from build123d import *

# Parameters (mm, degrees)
SKETCH1_W               = 22
SKETCH1_H               = 28
BOSS_EXTRUDE1_DEPTH     = 1.75
SKETCH2_R               = 1.3
SKETCH2_R_2             = 1
CUT_EXTRUDE1_DEPTH      = 18.890290663
SKETCH3_R               = 0.6
CUT_EXTRUDE2_DEPTH      = 18.890290663
LPATTERN1_COUNT         = 4
LPATTERN1_PITCH         = 2.54
MIRROR1_COPY_1_SKETCH_R = 0.6
MIRROR1_COPY_1_DEPTH    = 18.890290663
MIRROR1_COPY_2_SKETCH_R = 0.6
MIRROR1_COPY_2_DEPTH    = 18.890290663
MIRROR1_COPY_3_SKETCH_R = 0.6
MIRROR1_COPY_3_DEPTH    = 18.890290663
SKETCH4_W               = 5
SKETCH4_H               = 4.4
BOSS_EXTRUDE2_DEPTH     = 1.2


with BuildPart() as part:
    # Sketch1 → Boss-Extrude1 (new body)
    with BuildSketch(Plane.XY):
        Rectangle(SKETCH1_W, SKETCH1_H)
    extrude(amount=BOSS_EXTRUDE1_DEPTH)

    # Sketch2 → Cut-Extrude1 (cut, through all)
    with BuildSketch(Plane.XY.offset(1.75)):
        with Locations((-9, -1)):
            Circle(SKETCH2_R)
        with Locations((-9, -12)):
            Circle(SKETCH2_R)
        with Locations((9, -12)):
            Circle(SKETCH2_R)
        with Locations((9, -1)):
            Circle(SKETCH2_R)
        with Locations((0, -6.5)):
            Circle(SKETCH2_R_2)
    extrude(amount=-CUT_EXTRUDE1_DEPTH, mode=Mode.SUBTRACT)

    # Sketch3 → Cut-Extrude2 (cut, through all)
    with BuildSketch(Plane.XY.offset(1.75)):
        with Locations((-1.27, 12.73)):
            Circle(SKETCH3_R)
    cut_extrude2 = extrude(amount=-CUT_EXTRUDE2_DEPTH, mode=Mode.SUBTRACT)

    # LPattern1: Cut-Extrude2 ×4
    with Locations(*[(-i * LPATTERN1_PITCH, 0, 0) for i in range(1, LPATTERN1_COUNT)]):
        add(cut_extrude2, mode=Mode.SUBTRACT)

    # Mirror1: Cut-Extrude2 across plane
    add(cut_extrude2.mirror(Plane(origin=(0, 0, 0), x_dir=(0, 0, 1), z_dir=(1, 0, 0))), mode=Mode.SUBTRACT)

    # Mirror1 copy 1 sketch → Mirror1 copy 1 (cut, through all)
    with BuildSketch(Plane(origin=(2.54, 0, 1.75), x_dir=(-1, 0, 0), z_dir=(0, 0, 1))):
        with Locations((-1.27, -12.73)):
            Circle(MIRROR1_COPY_1_SKETCH_R)
    extrude(amount=-MIRROR1_COPY_1_DEPTH, mode=Mode.SUBTRACT)

    # Mirror1 copy 2 sketch → Mirror1 copy 2 (cut, through all)
    with BuildSketch(Plane(origin=(5.08, 0, 1.75), x_dir=(-1, 0, 0), z_dir=(0, 0, 1))):
        with Locations((-1.27, -12.73)):
            Circle(MIRROR1_COPY_2_SKETCH_R)
    extrude(amount=-MIRROR1_COPY_2_DEPTH, mode=Mode.SUBTRACT)

    # Mirror1 copy 3 sketch → Mirror1 copy 3 (cut, through all)
    with BuildSketch(Plane(origin=(7.62, 0, 1.75), x_dir=(-1, 0, 0), z_dir=(0, 0, 1))):
        with Locations((-1.27, -12.73)):
            Circle(MIRROR1_COPY_3_SKETCH_R)
    extrude(amount=-MIRROR1_COPY_3_DEPTH, mode=Mode.SUBTRACT)

    # Sketch4 → Boss-Extrude2 (add)
    with BuildSketch(Plane.XY.offset(1.75)):
        with Locations((0, -6.5)):
            Rectangle(SKETCH4_W, SKETCH4_H)
    extrude(amount=BOSS_EXTRUDE2_DEPTH)


solid = part.part
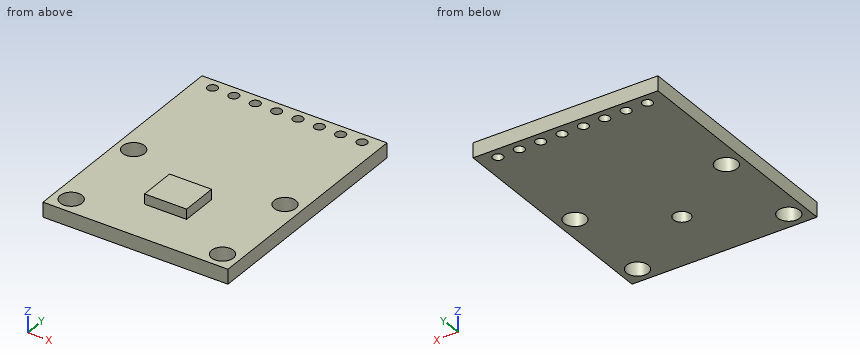
The model under review builds one solid part; all positions refer to its coordinate system, in mm. Give positions to 0.01 mm unless a question says otherwise; leave off trailing zeros. Loops run counter-clockwise (first coordinate to the right, second up) from the corner with the lowest first, then second, coordinate; pieces in that order, holes last. Notation, with made-up numbers: (61, 48) -> (114, 48) arc R25 ccw to (114, 85) -> close; hole circle Ø3 at (49, 74.25). An arc over 180 degrees is marked (long way). Put each result on its own line as item: value. Start each with the question number.
1. We need section D-D on x = -9. State the section outline as (y, z) points.
2. Wall thickness on probe 1 along Y at (x, z) = (9, 0.7); probe 2 along Z at (x, y) = (7.5, -6.5); probe 3 along Y at (x, z) = (1.5, 2.45): over which ranges is each line inside the solid? List them lowest first.
3. We need section C-C on y = -6.5. State the section outline as (x, z) points, then the cut area to 3 significant figures.
4. Clearance check with flat-ended pins moving along their axes: P1, Ø1.9, axis at x = 8.89, y = 12.73, coming from the +Z side; P2, Ø0.6, axis at x = 1, z = 2.5, coming from the +Y side. State where each tip first meets the part, or that it passes through.
5. We need section A-A on x = 6.35. State the section outline as (y, z) points, then the cut area to 3 significant figures.
6. We need section B-B on z = 0.7. State how many separate pieces and enclosed holes the cut face has, then the cut area to 3 significant figures.
Determined:
1. outline: (-14, 0) -> (-13.3, 0) -> (-13.3, 1.75) -> (-14, 1.75) -> close; (-10.7, 0) -> (-2.3, 0) -> (-2.3, 1.75) -> (-10.7, 1.75) -> close; (0.3, 0) -> (12.14, 0) -> (12.14, 1.75) -> (0.3, 1.75) -> close; (13.32, 0) -> (14, 0) -> (14, 1.75) -> (13.32, 1.75) -> close
2. probe 1: -14 to -13.3, -10.7 to -2.3, 0.3 to 12.14, 13.32 to 14
2. probe 2: 0 to 1.75
2. probe 3: -8.7 to -4.3
3. outline: (-11, 0) -> (-1, 0) -> (-1, 1.75) -> (1, 1.75) -> (1, 0) -> (11, 0) -> (11, 1.75) -> (2.5, 1.75) -> (2.5, 2.95) -> (-2.5, 2.95) -> (-2.5, 1.75) -> (-11, 1.75) -> close
3. area: 41.0 mm^2
4. P1: z = 1.75
4. P2: y = -4.3
5. outline: (-14, 0) -> (12.13, 0) -> (12.13, 1.75) -> (-14, 1.75) -> close; (13.33, 0) -> (14, 0) -> (14, 1.75) -> (13.33, 1.75) -> close
5. area: 46.9 mm^2
6. separate pieces: 1
6. enclosed holes: 13
6. area: 583 mm^2
